Here's how the part is built. I have some questions about the finished solid (model axes, mm). A direction names the side the tool comes from. Round coordinates to 2 decimals unless told otherwise and drop trailing zeros. Order: outer loops, then holes, each group sorted by start corner. A loop starts at its lowest first (then second) coordinate and runs counter-clockwise, first axis right, second up. Notation, with made-up numbers: M 11,4.5 L 21,4.5 A18 cw 21,30.5 Z; hole C 64.25,-2.75 d4. An arc over 180 degrees is marked long. Write item = value, one per line. Start each with the question number.
Item 1: Please list where these lines run through material, in increasing order: L1, parallel to X at y = 0, z = 3.5; L2, parallel to Z at x = -52.5, y = 45.5.
Item 2: We'd pull the mould along X, two halves only. Please class faces 1 (the face through (-67.5, -1, 5)), 2 (the face through (-62, 57.5, 14)), 3 (the face through (-57.5, 63, 14)): pulls with the +X half, pulls with the -X half, needs draft (parallel to the pull), parting line crosses it, or undercut.
Item 3: I want a section at C-C, the plane y = -18.5. List the corners of the cut face in (x, z) for me, plus the area to 3 significant figures.
Item 4: I want a section at B-B, the plane z = 14.25. List the corners of the cut face in (x, y) for me.
Item 5: I want a section at D-D, the plane z = 2.5. List the corners of the cut face in (x, y) for me.
Item 6: For faces 4 (the face through (-64, 0, 6)), 5 (the face through (57.5, 63, 14)), 6 (the face through (-62.44, -2.75, 3.45)), 7 (the face through (62, 57.5, 14)), which set-ups out of +Z, -Z, +X, -X, +Y, -Y let a thin tool reach every point of the face, with its end or its side?
Item 7: I want a section at A-A, the plane x = 0. List the corners of the cut face in (y, z) for me.
Item 8: I'm going to push a flat-ended pin straight in: P1, Ø1.5, axis at x = 43.5, z = 12, coming from the +Y side. Where does the tip first touch, or does it pass through?
Autodesk Inventor part; units mm, degrees
ref_plane "YZ Plane" through (0, 0, 0) normal (1, 0, 0) x (0, 1, 0)
ref_plane "XZ Plane" through (0, 0, 0) normal (0, 1, 0) x (-1, 0, 0)
ref_plane "XY Plane" through (0, 0, 0) normal (0, 0, 1) x (1, 0, 0)
sketch "Boceto1" plane through (0, 0, 0) normal (0, 0, 1) x (1, 0, 0)
  circle A0 centre (0, 0) radius 62.5
  line L0 (62.5, 0) -> (67.5, 0)
  line L1 (0, 62.5) -> (0, 67.5)
  line L2 (0, 62.5) -> (5, 62.5) construction
  line L3 (0, 67.5) -> (67.5, 67.5)
  line L4 (67.5, 67.5) -> (67.5, 0)
  line L5 (-62.5, 0) -> (-67.5, 0)
  line L6 (-62.5, 0) -> (-57.5, 0) construction
  line L7 (0, -62.5) -> (0, -67.5)
  line L8 (0, -62.5) -> (5, -62.5) construction
  line L9 (0, -67.5) -> (-67.5, -67.5)
  line L10 (-67.5, -67.5) -> (67.5, -67.5)
  line L11 (67.5, -67.5) -> (67.5, 67.5)
  line L12 (67.5, 67.5) -> (-67.5, 67.5)
  line L13 (-67.5, 67.5) -> (-67.5, -67.5)
  dimension "d0" = 125
  dimension "d1" = 5
  dimension "d2" = 5
  dimension "d3" = 90
  dimension "d4" = 90
  dimension "d5" = 5
  dimension "d6" = 180
  dimension "d7" = 5
  dimension "d8" = 90
  dimension "d9" = 90
extrude "Extrusión1" add sketch "Boceto1" along normal blind 7 contours L0 L11 L10 L7 A0 | A0 L1 L3 L4 L0 | A0 L5 L13 L12 L1 | L7 L9 L13 L5 A0
sketch "Boceto2" plane through (0, 0, 7) normal (0, 0, 1) x (1, 0, 0)
  line L0 (-67.5, 67.5) -> (67.5, 67.5)
  line L1 (67.5, 67.5) -> (67.5, -67.5)
  line L2 (67.5, -67.5) -> (-67.5, -67.5)
  line L3 (-67.5, -67.5) -> (-67.5, 67.5)
  circle A0 centre (0, 0) radius 58.5
  dimension "d12" = 117
extrude "Extrusión2" add sketch "Boceto2" along normal blind 3
sketch "Boceto3" plane through (0, 0, 10) normal (0, 0, 1) x (1, 0, 0)
  line L0 (-67.5, -67.5) -> (-57.5, -67.5)
  line L1 (-57.5, -67.5) -> (-57.5, -57.5)
  line L2 (-57.5, -57.5) -> (-67.5, -57.5)
  line L3 (-67.5, -57.5) -> (-67.5, -67.5)
  line L4 (67.5, 67.5) -> (57.5, 67.5)
  line L5 (57.5, 67.5) -> (57.5, 57.5)
  line L6 (57.5, 57.5) -> (67.5, 57.5)
  line L7 (67.5, 57.5) -> (67.5, 67.5)
  line L8 (-67.5, 67.5) -> (-57.5, 67.5)
  line L9 (-57.5, 67.5) -> (-57.5, 57.5)
  line L10 (-57.5, 57.5) -> (-67.5, 57.5)
  line L11 (-67.5, 57.5) -> (-67.5, 67.5)
  line L12 (67.5, -67.5) -> (57.5, -67.5)
  line L13 (57.5, -67.5) -> (57.5, -57.5)
  line L14 (57.5, -57.5) -> (67.5, -57.5)
  line L15 (67.5, -57.5) -> (67.5, -67.5)
  point P0 (0, 0)
  dimension "d15" = 10
  dimension "d16" = 10
  dimension "d17" = 10
  dimension "d18" = 10
  dimension "d19" = 10
  dimension "d20" = 10
  dimension "d21" = 10
  dimension "d22" = 10
extrude "Extrusión3" add sketch "Boceto3" along normal blind 8
sketch "Boceto4" plane through (-67.5, -67.5, 0) normal (-1, 0, 0) x (0, 0, 1)
  line L0 (0, 67.5) -> (10, 67.5)
  line L1 (10, 10) -> (10, 125)
  line L2 (10, 67.5) -> (10, 71.5)
  line L3 (10, 67.5) -> (14, 67.5) construction
  line L4 (10, 67.5) -> (10, 63.5)
  line L5 (10, 67.5) -> (14, 67.5) construction
  line L6 (10, 67.5) -> (6, 67.5)
  arc A0 (10, 71.5) -> (10, 63.5) centre (10, 67.5) ccw
  dimension "d25" = 4
  dimension "d26" = 90
  dimension "d27" = 4
  dimension "d28" = 90
  dimension "d29" = 4
extrude "Extrusión4" cut sketch "Boceto4" against normal blind 10
properties part number "lamp_holder_v1"
Filled in:
q1.L1 = -67.5 to -62.5, 62.5 to 67.5
q1.L2 = 0 to 10
q2.face_1 = pulls with the -X half
q2.face_2 = needs draft
q2.face_3 = undercut
q3.outline = M -67.5,0 L -59.7,0 L -59.7,7 L -55.5,7 L -55.5,10 L -67.5,10 Z; M 55.5,7 L 59.7,7 L 59.7,0 L 67.5,0 L 67.5,10 L 55.5,10 Z
q3.area = 181 mm^2
q4.outline = M -67.5,-67.5 L -57.5,-67.5 L -57.5,-57.5 L -67.5,-57.5 Z; M -67.5,57.5 L -57.5,57.5 L -57.5,67.5 L -67.5,67.5 Z; M 57.5,-67.5 L 67.5,-67.5 L 67.5,-57.5 L 57.5,-57.5 Z; M 57.5,57.5 L 67.5,57.5 L 67.5,67.5 L 57.5,67.5 Z
q5.outline = M -67.5,-67.5 L 67.5,-67.5 L 67.5,67.5 L -67.5,67.5 Z; hole C 0,0 d125
q6.face_4 = +Z, -X
q6.face_5 = +Z, +Y, -Y
q6.face_6 = -Z
q6.face_7 = +Z, +X, -X
q7.outline = M -67.5,0 L -62.5,0 L -62.5,7 L -58.5,7 L -58.5,10 L -67.5,10 Z; M 58.5,7 L 62.5,7 L 62.5,0 L 67.5,0 L 67.5,10 L 58.5,10 Z
q8.P1 = through
